```python
from build123d import *

# Parameters (mm, degrees)
F0_W = 1
F0_H = 7


with BuildPart() as f1:
    # F0 (on Right) → F1 (revolve)
    with BuildSketch(Plane.YZ):
        Polygon((0, 10), (0, 8.5), (1, 8.5), (1.5, 8.5), (1.5, 10), align=None)
        with Locations((0.5, 5)):
            Rectangle(F0_W, F0_H)
        Polygon((0, 1.5), (0, 0), (2, 0), (2, 1.5), (1, 1.5), align=None)
    revolve(axis=Axis((0, 1, 0), (0, 1, 0)))


solid = f1.part
```
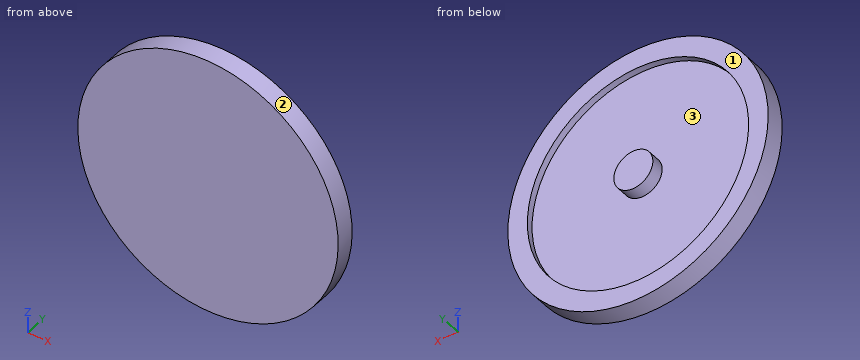
Read the model definition and answer for the solid it produces. Units are mm, in the model's axes. Face numbers are marked on the shaded views. Give positions to 0.01 mm unless a question says otherwise; leave off trailing zeros. Write each loop counter-clockwise with the first axis right and the second up, starting at its lowest first coordinate (ties: lowest second). Pieces come first, ordered by that corner, then holes. Notation, with made-up numbers: (68.5, 77.25) - (114.5, 77.25) arc R35 ccw to (114.5, 112.25) - close; hole circle Ø7 at (22.5, 14.5). An arc over 180 degrees is marked (long way). Write item = value, one per line. Start each with the question number.
Item 1: Find section B-B (x = 0). Give the vertices of the cut face in (y, z), then the cut area to 3 significant figures.
Item 2: Find section C-C (z = 4). Give the vertices of the cut face in (x, y).
Item 3: Find section A-A (z = 0). Give the vertices of the cut face in (x, y).
Item 4: Find section D-D (x = -5.25). Give the vertices of the cut face in (y, z).
Item 5: The mould has two halves that part along X. Classify the marked faces 1, 2 and 3: +X half, -X half, draft (parallel to the pull), parting line (faces both ways), or undercut.
Item 6: Each of these flat-tipped pins is pushed along its axis until it touches: P1, Ø2, axis at x = -0.5, z = -2.5, coming from the +Y side; P2, Ø6, axis at x = -5.5, z = -6.5, coming from the +Y side. Where does it stop, or does it pass through?
Item 7: Find the intervals of material crossed by probe 1 along X at (y, z) = (1.4, 0); probe 2 along Y at (x, z) = (-2, 5.75); probe 3 along Y at (x, z) = (7.75, -6), in increasing order. Write a range as [from, to].
Response:
q1.outline = (0, -10) - (1.5, -10) - (1.5, -8.5) - (1, -8.5) - (1, -1.5) - (2, -1.5) - (2, 1.5) - (1, 1.5) - (1, 8.5) - (1.5, 8.5) - (1.5, 10) - (0, 10) - close
q1.area = 24.5 mm²
q2.outline = (-9.17, 0) - (9.17, 0) - (9.17, 1.5) - (7.5, 1.5) - (7.5, 1) - (-7.5, 1) - (-7.5, 1.5) - (-9.17, 1.5) - close
q3.outline = (-10, 0) - (10, 0) - (10, 1.5) - (8.5, 1.5) - (8.5, 1) - (1.5, 1) - (1.5, 2) - (-1.5, 2) - (-1.5, 1) - (-8.5, 1) - (-8.5, 1.5) - (-10, 1.5) - close
q4.outline = (0, -8.51) - (1.5, -8.51) - (1.5, -6.68) - (1, -6.68) - (1, 6.68) - (1.5, 6.68) - (1.5, 8.51) - (0, 8.51) - close
q5.face_1 = draft
q5.face_2 = parting line
q5.face_3 = undercut
q6.P1 = 1
q6.P2 = 1.5
q7.probe_1 = [-10, -8.5], [-1.5, 1.5], [8.5, 10]
q7.probe_2 = [0, 1]
q7.probe_3 = [0, 1.5]
